```python
from build123d import *

# Parameters (mm, degrees)
SKETCH1_W                = 8
SKETCH1_H                = 8
BOSS_EXTRUDE1_DEPTH      = 3.2
SKETCH2_R                = 2.4
BOSS_EXTRUDE2_DEPTH      = 1.8
SKETCH3_W                = 4.8
SKETCH3_H                = 4.8
CUT_EXTRUDE1_DEPTH       = 1.8
BOSS_EXTRUDE3_DEPTH      = 1.6
BOSS_EXTRUDE3_DEPTH_BACK = 1.6


with BuildPart() as part:
    # Sketch1 → Boss-Extrude1 (new body)
    with BuildSketch(Plane(origin=(0, 0, 0), x_dir=(1, 0, 0), z_dir=(0, 1, 0))):
        with Locations((4, 4)):
            Rectangle(SKETCH1_W, SKETCH1_H)
    extrude(amount=BOSS_EXTRUDE1_DEPTH)

    # Sketch2 → Boss-Extrude2 (add)
    with BuildSketch(Plane(origin=(0, 3.2, 0), x_dir=(1, 0, 0), z_dir=(0, 1, 0))):
        with Locations(Location((4, 4, 0), (0, 0, 270))):
            Circle(SKETCH2_R)
    extrude(amount=BOSS_EXTRUDE2_DEPTH)

    # Sketch3 → Cut-Extrude1 (cut)
    with BuildSketch(Plane.XZ):
        with Locations((4, -4)):
            Rectangle(SKETCH3_W, SKETCH3_H)
    extrude(amount=-CUT_EXTRUDE1_DEPTH, mode=Mode.SUBTRACT)

    # Sketch4 → Boss-Extrude3 (add, two sides: drawn at the far end of the back side and taken through both)
    with BuildSketch(Plane(origin=(0, 0, -4), x_dir=(-1, 0, 0), z_dir=(0, 0, -1)).offset(-BOSS_EXTRUDE3_DEPTH_BACK)):
        with BuildLine():
            Line((-8, 3.2), (-9.91253312, 3.2))
            ThreePointArc((-9.91253312, 3.2), (-11.093178218, 4.86443349), (-13.065366807, 5.388584094))
            ThreePointArc((-13.065366807, 5.388584094), (-13.747146024, 4.576071264), (-12.934633193, 3.894292047))
            ThreePointArc((-12.934633193, 3.894292047), (-11.303899579, 2.4), (-12.934633193, 0.905707953))
            ThreePointArc((-12.934633193, 0.905707953), (-13.747146024, 0.223928736), (-13.065366807, -0.588584094))
            ThreePointArc((-13.065366807, -0.588584094), (-11.98026217, -0.48472207), (-11.003899579, 0))
            Line((-11.003899579, 0), (-8, 0))
            Line((-8, 0), (-8, 3.2))
        make_face()
    extrude(amount=BOSS_EXTRUDE3_DEPTH + BOSS_EXTRUDE3_DEPTH_BACK)


solid = part.part
```
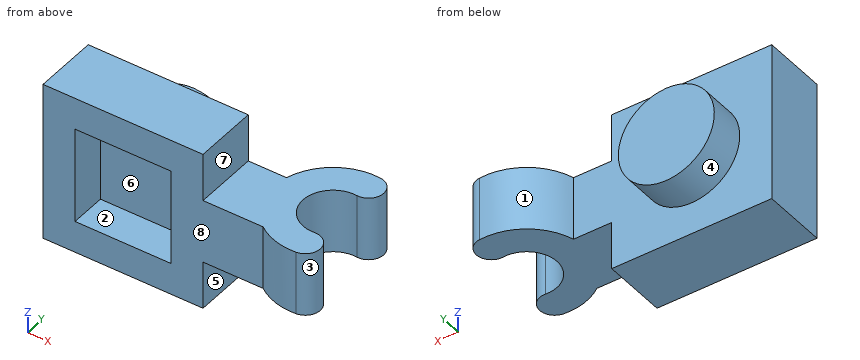
Check sheet for the modelled part. Datum: model origin and axes. Units: mm. Face numbers are marked on the shaded views. A direction names the side the tool comes from. Give positions to 0.01 mm unless a question says otherwise; leave off trailing zeros. Write each loop counter-clockwise with the first axis right and the second up, starting at its lowest first coordinate (ties: lowest second). Pieces come first, ordered by that corner, then holes.
Item 1: Draft check along Y on the marked faces 1, 2 and 3. Enter one of: released by +Y, released by -Y, zero draft, split by the parting line, or undercut.
Item 2: Cross-section at A-A (x = 12). Enter the section's corners in (y, z).
Item 3: Cross-section at B-B (y = 4.45). Enter the section's corners in (x, z), and give its area (3 significant figures).
Item 4: Scan lines: L1, parallel to X at y = 0.2, z = -2.5; L2, parallel to Z at x = 4.25, y = 1.2; L3, parallel to X at y = 0.5, z = -2. Record each from-to range of solid material in increasing order.
Item 5: Cross-section at D-D (x = 4). Enter the section's corners in (y, z), and give its area (3 significant figures).
Item 6: Gauge pin test, flat ends, axial feed: pin 1 (1.4 mm diameter, centred on x = 4.5, z = -4, fed in from +Y); pin 2 (1.2 mm diameter, centred on y = 2, z = -1, fed in from +X); pin 3 (1.7 mm diameter, centred on x = 11.5, y = 1, fed in from +Z). Record the tip position at first contact, or that the pin passes through.
Item 7: Access from +Z, -Z, +X, -X, +Y, -Y to the whole of each face (thin tool, end or side, straight path). Record for the marked faces 4, 5, 6, 7 and 8.
Item 8: Cross-section at C-C (z = -4). Enter the section's corners in (x, y).
Report:
1. face 1: released by +Y
1. face 2: zero draft
1. face 3: undercut
2. outline: (-0.49, -5.6) - (1.13, -5.6) - (1.13, -2.4) - (-0.49, -2.4) - close; (3.67, -5.6) - (5.29, -5.6) - (5.29, -2.4) - (3.67, -2.4) - close
3. outline: circle Ø4.8 at (4, -4); (10.61, -5.6) - (13.73, -5.6) - (13.73, -2.4) - (10.61, -2.4) - close
3. area: 28.1 mm2
4. L1: x = 0 to 1.6, 6.4 to 13.75
4. L2: z = -8 to -6.4, -1.6 to 0
4. L3: x = 0 to 1.6, 6.4 to 8
5. outline: (0, -8) - (3.2, -8) - (3.2, -6.4) - (5, -6.4) - (5, -1.6) - (3.2, -1.6) - (3.2, 0) - (0, 0) - (0, -1.6) - (1.8, -1.6) - (1.8, -6.4) - (0, -6.4) - close
5. area: 25.6 mm2
6. pin 1: stops at y = 5
6. pin 2: stops at x = 8
6. pin 3: stops at z = -2.4
7. face 4: +Y
7. face 5: -Z, +X, +Y, -Y
7. face 6: -Y
7. face 7: +Z, +X, +Y, -Y
7. face 8: +Z, -Z, -X, -Y
8. outline: (0, 0) - (1.6, 0) - (1.6, 1.8) - (6.4, 1.8) - (6.4, 0) - (11, 0) arc R3 ccw to (13.07, -0.59) arc R0.75 ccw to (12.93, 0.91) arc R1.5 cw (long way) to (12.93, 3.89) arc R0.75 ccw to (13.07, 5.39) arc R3 ccw to (9.91, 3.2) - (6.4, 3.2) - (6.4, 5) - (1.6, 5) - (1.6, 3.2) - (0, 3.2) - close
